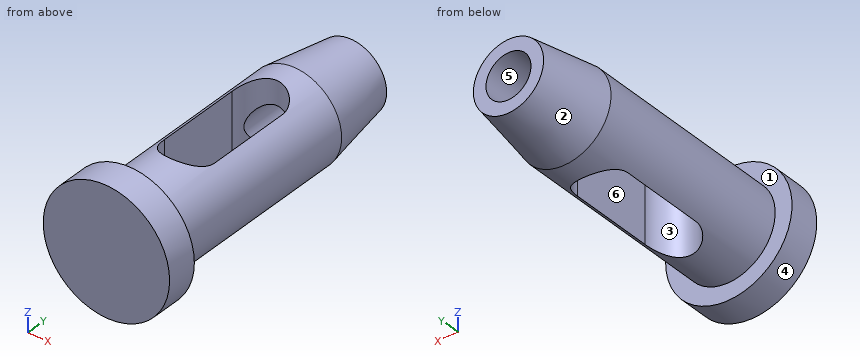
from build123d import *

# Parameters (mm, degrees)
CUT_EXTRUDE1_DEPTH      = 23.5
CUT_EXTRUDE1_DEPTH_BACK = 23.5
CUT_EXTRUDE2_REACH      = 111
SKETCH3_R               = 8


with BuildPart() as part:
    # Sketch1 → Revolve1 (revolve)
    with BuildSketch(Plane.XY):
        Polygon((0, 0), (22.5, 0), (22.5, 11), (16.5, 11), (16.5, 84), (12.5, 109), (0, 109), align=None)
    revolve(axis=Axis((0, 0, 0), (0, 1, 0)))

    # Sketch2 → Cut-Extrude1 (cut, two sides)
    with BuildSketch(Plane.XY) as cut_extrude1_sk:
        with BuildLine():
            Line((9, 67), (9, 37))
            ThreePointArc((9, 37), (0, 28), (-9, 37))
            Line((-9, 37), (-9, 67))
            ThreePointArc((-9, 67), (0, 76), (9, 67))
        make_face()
    extrude(amount=CUT_EXTRUDE1_DEPTH, mode=Mode.SUBTRACT)
    extrude(cut_extrude1_sk.sketch, amount=-CUT_EXTRUDE1_DEPTH_BACK, mode=Mode.SUBTRACT)

    # Sketch3 → Cut-Extrude2 (cut, up to next)
    with BuildSketch(Plane(origin=(0, 109, 0), x_dir=(1, 0, 0), z_dir=(0, 1, 0)), mode=Mode.PRIVATE) as cut_extrude2_sk1:
        Circle(SKETCH3_R)
    cut_extrude2_tool1 = extrude(cut_extrude2_sk1.sketch, amount=-CUT_EXTRUDE2_REACH, mode=Mode.PRIVATE) & part.part
    add(cut_extrude2_tool1.solids().sort_by_distance((0, 109, 0))[0], mode=Mode.SUBTRACT)


solid = part.part
CAD build for the part. Positions are in the model's coordinates, mm. Face numbers are marked on the shaded views. A direction names the side the tool comes from. Round coordinates to 2 decimals unless told otherwise and drop trailing zeros. Write each loop counter-clockwise with the first axis right and the second up, starting at its lowest first coordinate (ties: lowest second). Pieces come first, ordered by that corner, then holes. Notation, with made-up numbers: M -11,25 L 3,25 A19 ccw 3,60 Z; hole C -20.5,-17 d1. An arc over 180 degrees is marked long. Use a Markdown table: item, result. Add a question column.
1. Drill centre lines: probe 1 along Z at (x, y) = (0, 81); probe 2 along Y at (x, z) = (16, 6); probe 3 along Y at (x, z) = (-5, 10.5). Where is each one in solid material? Low to high.
2. Pull direction X, two halves, no side cores. Call the marked faces 1, 2 and 3: released by +X, released by -X, zero draft, split by the parting line, or undercut.
3. Slice it at B-B on z = 0. Give the cut face in (x, y), then the cut area to 3 significant figures.
4. 3-axis set-ups, long thin cutter, end or side, ignore diameter. For the marked faces 4, 5 and 6: which of +Z, -Z, +X, -X, +Y, -Y reach the whole face in a straight line?
5. Slice it at C-C on y = 97. Give the cut face in (x, z).
6. Flat gauge pins, fed straight in: P1, Ø5, axis at x = 10, y = 61.5, coming from the -Z side; P2, Ø2, axis at y = 84.5, z = 6, coming from the +X side; P3, Ø10, axis at x = 9.5, y = 29.5, coming from the +Z side. Where does each tip first touch, or does it go through?
7. Slice it at D-D on x = 19. Give the cut face in (y, z), then the cut area to 3 significant figures.
8. Slice it at A-A on x = 0. Give the cut face in (y, z).
Reply:
| question | item | result |
|---|---|---|
| 1 | probe 1 | z = -16.5 to -8, 8 to 16.5 |
| 1 | probe 2 | y = 0 to 11 |
| 1 | probe 3 | y = 0 to 29.52, 74.48 to 109 |
| 2 | face 1 | zero draft |
| 2 | face 2 | split by the parting line |
| 2 | face 3 | undercut |
| 3 | outline | M -22.5,0 L 22.5,0 L 22.5,11 L 16.5,11 L 16.5,84 L 12.5,109 L 8,109 L 8,71.12 A9 cw 9,67 L 9,37 A9 cw -9,37 L -9,67 A9 cw -8,71.12 L -8,109 L -12.5,109 L -16.5,84 L -16.5,11 L -22.5,11 Z |
| 3 | area | 2,280 mm^2 |
| 4 | face 4 | +Y, -Y |
| 4 | face 5 | +Y |
| 4 | face 6 | +Z, -Z |
| 5 | outline | C 0,0 d28.84; hole C 0,0 d16 |
| 6 | P1 | stops at z = -13.83 |
| 6 | P2 | stops at x = 15.68 |
| 6 | P3 | stops at z = 15.87 |
| 7 | outline | M 0,-12.05 L 11,-12.05 L 11,12.05 L 0,12.05 Z |
| 7 | area | 265 mm^2 |
| 8 | outline | M 0,-22.5 L 11,-22.5 L 11,-16.5 L 28,-16.5 L 28,16.5 L 11,16.5 L 11,22.5 L 0,22.5 Z; M 76,-16.5 L 84,-16.5 L 109,-12.5 L 109,-8 L 76,-8 Z; M 76,8 L 109,8 L 109,12.5 L 84,16.5 L 76,16.5 Z |
